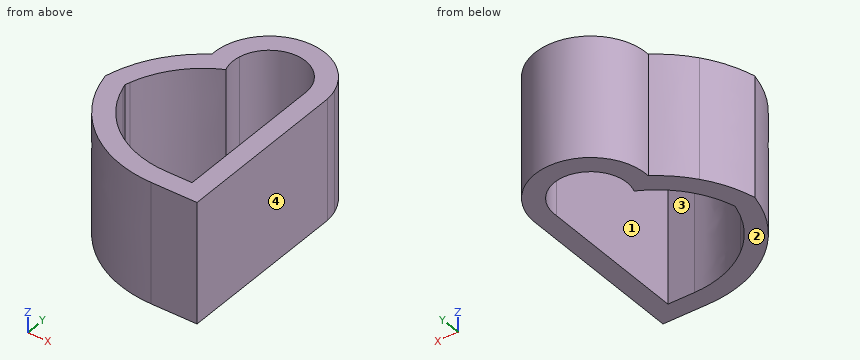
from build123d import *

# Parameters (mm, degrees)
BOSS_EXTRUDE1_DEPTH = 5


with BuildPart() as part:
    # Sketch1 → Boss-Extrude1 (new body)
    with BuildSketch(Plane.XY):
        with BuildLine():
            ThreePointArc((-75.265428178, 20.9), (-75.130279043, 20.511046865), (-75.105982855, 20.1))
            Line((-75.105982855, 20.1), (-75.105982855, 19.853719883))
            add(Edge.make_bspline(
                [(-74.305982855, 19.570019979), (-74.57545788, 19.689791559), (-74.842109989, 19.784227542), (-75.105982855, 19.853719883)],
                knots=[-0.347916047, -0.347916047, -0.347916047, -0.347916047, -0.203467167, -0.203467167, -0.203467167, -0.203467167], degree=3))
            Line((-74.305982855, 19.570019979), (-74.305982855, 20.071878785))
            Line((-74.305982855, 20.071878785), (-74.305982855, 20.363828129))
            ThreePointArc((-74.305982855, 20.363828129), (-74.339463682, 20.634853388), (-74.404831342, 20.9))
            Line((-74.404831342, 20.9), (-75.265428178, 20.9))
        make_face()
        with BuildLine():
            add(Edge.make_bspline(
                [(-74.305982855, 19.570019979), (-74.57545788, 19.689791559), (-74.842109989, 19.784227542), (-75.105982855, 19.853719883)],
                knots=[-0.347916047, -0.347916047, -0.347916047, -0.347916047, -0.203467167, -0.203467167, -0.203467167, -0.203467167], degree=3))
            Line((-75.105982855, 19.853719883), (-75.105982855, 16.984329869))
            Line((-75.105982855, 16.984329869), (-75.105982855, 14.140403881))
            add(Edge.make_bspline(
                [(-75.105982855, 14.140403881), (-74.843255413, 14.206157854), (-74.576591527, 14.295030515), (-74.305982855, 14.407070854)],
                knots=[1.201768628, 1.201768628, 1.201768628, 1.201768628, 1.343435707, 1.343435707, 1.343435707, 1.343435707], degree=3))
            Line((-74.305982855, 14.407070854), (-74.305982855, 17.699135935))
            Line((-74.305982855, 17.699135935), (-74.305982855, 19.570019979))
        make_face()
        with BuildLine():
            ThreePointArc((-78.067947351, 20.532623393), (-76.79630986, 21.70512917), (-75.265428178, 20.9))
            Line((-75.265428178, 20.9), (-74.404831342, 20.9))
            ThreePointArc((-74.404831342, 20.9), (-77.006960237, 22.481805089), (-78.898061562, 20.094983372))
            add(Edge.make_bspline(
                [(-78.067947351, 20.532623393), (-78.358359688, 20.413646492), (-78.636457372, 20.266940111), (-78.898061562, 20.094983372)],
                knots=[0.295059063, 0.295059063, 0.295059063, 0.295059063, 0.440738585, 0.440738585, 0.440738585, 0.440738585], degree=3))
        make_face()
        with BuildLine():
            add(Edge.make_bspline(
                [(-78.003515184, 19.685010862), (-78.104869219, 19.63560007), (-78.355344555, 19.500363503), (-78.967656438, 19.082169769), (-79.659987233, 18.331266584), (-80.013929538, 17.564650836), (-80.12711921, 17.200243393)],
                knots=[0.344074201, 0.344074201, 0.344074201, 0.344074201, 0.406881084, 0.502455065, 0.753682598, 0.966213979, 0.966213979, 0.966213979, 0.966213979], degree=3))
            ThreePointArc((-78.003515184, 19.685010862), (-78.097030736, 20.104157384), (-78.067947351, 20.532623393))
            add(Edge.make_bspline(
                [(-78.067947351, 20.532623393), (-78.358359688, 20.413646492), (-78.636457372, 20.266940111), (-78.898061562, 20.094983372)],
                knots=[0.295059063, 0.295059063, 0.295059063, 0.295059063, 0.440738585, 0.440738585, 0.440738585, 0.440738585], degree=3))
            add(Edge.make_bspline(
                [(-78.898061562, 20.094983372), (-79.044158498, 19.998951452), (-79.506474474, 19.658143157), (-79.905620688, 19.237259361), (-80.14350503, 18.917192132)],
                knots=[0.440738585, 0.440738585, 0.440738585, 0.440738585, 0.522095585, 0.707584074, 0.707584074, 0.707584074, 0.707584074], degree=3))
            add(Edge.make_bspline(
                [(-80.143505006, 18.917192121), (-80.243393446, 18.301629507), (-80.235757559, 17.730205674), (-80.12711921, 17.200243393)],
                knots=[-0.342301016, -0.342301016, -0.342301016, -0.342301016, -0.038630201, -0.038630201, -0.038630201, -0.038630201], degree=3))
        make_face()
        with BuildLine():
            add(Edge.make_bspline(
                [(-80.12711921, 17.200243393), (-80.147727954, 17.133894765), (-80.166711829, 17.067112434), (-80.184053986, 17)],
                knots=[0.966213979, 0.966213979, 0.966213979, 0.966213979, 1.00491013, 1.00491013, 1.00491013, 1.00491013], degree=3))
            add(Edge.make_bspline(
                [(-80.143505006, 18.917192121), (-80.243393446, 18.301629507), (-80.235757559, 17.730205674), (-80.12711921, 17.200243393)],
                knots=[-0.342301016, -0.342301016, -0.342301016, -0.342301016, -0.038630201, -0.038630201, -0.038630201, -0.038630201], degree=3))
            add(Edge.make_bspline(
                [(-80.14350503, 18.917192132), (-80.240407946, 18.786811765), (-80.486796547, 18.418759671), (-80.740911848, 17.89685783), (-80.901091234, 17.421401242), (-80.969166274, 17.159575272), (-80.996010355, 17.055421709), (-81.010331575, 17)],
                knots=[0.707584074, 0.707584074, 0.707584074, 0.707584074, 0.783143378, 0.913667274, 0.978929222, 1.011560196, 1.044191171, 1.044191171, 1.044191171, 1.044191171], degree=3))
            add(Edge.make_bspline(
                [(-81.010331575, 17), (-80.995912214, 16.944198497), (-80.968881368, 16.839270604), (-80.900356676, 16.576013924), (-80.741671714, 16.105170367), (-80.311695813, 15.221571956), (-79.37871474, 14.137722448), (-77.891914282, 13.2952625), (-76.763881291, 13.1), (-76.204616771, 13.1)],
                knots=[-0.043877202, -0.043877202, -0.043877202, -0.043877202, -0.011256039, 0.021365123, 0.086607448, 0.217092099, 0.478061399, 0.7390307, 1, 1, 1, 1], degree=3))
            Line((-76.204616771, 13.1), (-74.305982855, 13.1))
            Line((-74.305982855, 13.1), (-74.305982855, 14.407070854))
            add(Edge.make_bspline(
                [(-75.105982855, 14.140403881), (-74.843255413, 14.206157854), (-74.576591527, 14.295030515), (-74.305982855, 14.407070854)],
                knots=[1.201768628, 1.201768628, 1.201768628, 1.201768628, 1.343435707, 1.343435707, 1.343435707, 1.343435707], degree=3))
            Line((-75.105982855, 14.140403881), (-75.105982855, 13.9))
            Line((-75.105982855, 13.9), (-76.204616771, 13.9))
            add(Edge.make_bspline(
                [(-78.772417568, 14.802007342), (-78.757445413, 14.790011818), (-78.387128598, 14.497563572), (-77.563800223, 14.051022081), (-76.655306258, 13.9), (-76.204616771, 13.9)],
                knots=[0.48691566, 0.48691566, 0.48691566, 0.48691566, 0.497562378, 0.748781189, 1, 1, 1, 1], degree=3))
            add(Edge.make_bspline(
                [(-80.126958505, 16.799254372), (-80.350350695, 15.691334532), (-80.041454579, 14.614718165), (-78.772417566, 14.802007352)],
                knots=[1.039358775, 1.039358775, 1.039358775, 1.039358775, 1.69125552, 1.69125552, 1.69125552, 1.69125552], degree=3))
            add(Edge.make_bspline(
                [(-80.184053986, 17), (-80.166668157, 16.932718561), (-80.147630382, 16.865768509), (-80.126958505, 16.799254372)],
                knots=[-0.004875245, -0.004875245, -0.004875245, -0.004875245, 0.033874117, 0.033874117, 0.033874117, 0.033874117], degree=3))
        make_face()
        with BuildLine():
            add(Edge.make_bspline(
                [(-80.126958505, 16.799254372), (-80.01361103, 16.434545856), (-79.667166625, 15.684835242), (-79.110726777, 15.07305693), (-78.772417568, 14.802007342)],
                knots=[0.033874117, 0.033874117, 0.033874117, 0.033874117, 0.246343567, 0.48691566, 0.48691566, 0.48691566, 0.48691566], degree=3))
            add(Edge.make_bspline(
                [(-80.126958505, 16.799254372), (-80.350350695, 15.691334532), (-80.041454579, 14.614718165), (-78.772417566, 14.802007352)],
                knots=[1.039358775, 1.039358775, 1.039358775, 1.039358775, 1.69125552, 1.69125552, 1.69125552, 1.69125552], degree=3))
        make_face()
    extrude(amount=BOSS_EXTRUDE1_DEPTH)


solid = part.part
Input: part model. Units: mm. Frame: model coordinates. Face numbers are marked on the shaded views. Coordinates: 2 decimals unless noted, no trailing zeros. Loops run counter-clockwise (first coordinate to the right, second up) from the corner with the lowest first, then second, coordinate; pieces in that order, holes last.
Q1. Draft query along X for the marked faces 1, 2, 3 and 4. Return one class per face: +X half, -X half, draft (parallel to the pull), parting line (faces both ways), or undercut.
Q2. Contact query for flat-ended pins moving along their axis: pin 1 (3 mm diameter, centred on x = -77.5, z = 1, fed in from +Y); pin 2 (1.5 mm diameter, centred on y = 20.5, z = 2.5, fed in from -X). Output: stop coordinate, or through.
Q3. Cut plane A-A (x = -75). Output: boundary loops of the cut face in (y, z).
Q4. Material intervals for line 1 (Y direction, x = -78.25, z = 1.95); line 2 (Y direction, x = -76.5, z = 1.5); line 3 (X direction, y = 16.75, z = 0.2), sorted ascending.
Working result:
1. face 1: undercut
1. face 2: draft
1. face 3: undercut
1. face 4: +X half
2. pin 1: stops at y = 22.52
2. pin 2: stops at x = -79.36
3. outline: (13.1, 0) - (21.87, 0) - (21.87, 5) - (13.1, 5) - close
4. line 1: y = 13.55 to 14.45, 19.55 to 21.82
4. line 2: y = 13.11 to 13.91, 21.71 to 22.52
4. line 3: x = -80.95 to -80.11, -75.11 to -74.31
